Check sheet for the modelled part. Datum: model origin and axes. Units: mm. Round coordinates to 2 decimals unless told otherwise and drop trailing zeros. Write each loop counter-clockwise with the first axis right and the second up, starting at its lowest first coordinate (ties: lowest second). Pieces come first, ordered by that corner, then holes. Notation, with made-up numbers: (60, 69) - (98, 69) arc R26 ccw to (98, 101) - close; hole circle Ø5 at (17.5, 58.25). An arc over 180 degrees is marked (long way). Use one line per item in the form item = value. Start each with the question number.
1) Section check B-B (y = 1). Count the separate pieces of the cut face and the enclosed holes in it, then the cut area to 3 significant figures.
2) Scan lines: probe 1 along X at (y, z) = (2.8, 0); probe 2 along X at (y, z) = (4.25, 62); probe 3 along Z at (x, y) = (-38, 2.1). Record each from-to range of solid material in increasing order.
3) Section check A-A (z = -107). Record the boundary of the cut face in (x, y).
4) Gauge pin test, flat end, axial feed: P1, Ø3, axis at x = 27.5, z = -36, coming from the -Y side. Record the tip position at first contact, or that the pin passes through.
from build123d import *

# Parameters (mm, degrees)
SKETCH1_W           = 300
SKETCH1_H           = 300
BOSS_EXTRUDE1_DEPTH = 4.5
SKETCH3_W           = 4.9
SKETCH3_H           = 15.4
CUT_EXTRUDE1_DEPTH  = 213.179758695
SKETCH6_W           = 15
SKETCH6_H           = 25
CUT_EXTRUDE2_DEPTH  = 213.179758695
SKETCH7_W           = 4.9
SKETCH7_H           = 10.4
CUT_EXTRUDE3_DEPTH  = 213.179758695
SKETCH8_R           = 1.55
CUT_EXTRUDE4_DEPTH  = 213.179758695
FILLET1_R           = 5


with BuildPart() as part:
    # Sketch1 → Boss-Extrude1 (new body)
    with BuildSketch(Plane(origin=(0, 0, 0), x_dir=(1, 0, 0), z_dir=(0, 1, 0))):
        Rectangle(SKETCH1_W, SKETCH1_H)
    extrude(amount=BOSS_EXTRUDE1_DEPTH)

    # Sketch3 → Cut-Extrude1 (cut, through all)
    with BuildSketch(Plane.XZ):
        with Locations((18.5, -130.5)):
            Rectangle(SKETCH3_W, SKETCH3_H)
        with Locations((18.5, -110.5)):
            Rectangle(SKETCH3_W, SKETCH3_H)
        with Locations((-18.5, -110.5)):
            Rectangle(SKETCH3_W, SKETCH3_H)
        with Locations((-18.5, -130.5)):
            Rectangle(SKETCH3_W, SKETCH3_H)
    extrude(amount=-CUT_EXTRUDE1_DEPTH, mode=Mode.SUBTRACT)

    # Sketch6 → Cut-Extrude2 (cut, through all)
    with BuildSketch(Plane.XZ):
        with Locations((37.5, -72.5)):
            Rectangle(SKETCH6_W, SKETCH6_H)
        with Locations((37.5, 72.5)):
            Rectangle(SKETCH6_W, SKETCH6_H)
        with Locations((-37.5, 72.5)):
            Rectangle(SKETCH6_W, SKETCH6_H)
        with Locations((-37.5, -72.5)):
            Rectangle(SKETCH6_W, SKETCH6_H)
    extrude(amount=-CUT_EXTRUDE2_DEPTH, mode=Mode.SUBTRACT)

    # Sketch7 → Cut-Extrude3 (cut, through all)
    with BuildSketch(Plane.XZ):
        with Locations((14, 130)):
            Rectangle(SKETCH7_W, SKETCH7_H)
        with Locations((-14, 130)):
            Rectangle(SKETCH7_W, SKETCH7_H)
        with Locations((-14, 115)):
            Rectangle(SKETCH7_W, SKETCH7_H)
        with Locations((14, 115)):
            Rectangle(SKETCH7_W, SKETCH7_H)
    extrude(amount=-CUT_EXTRUDE3_DEPTH, mode=Mode.SUBTRACT)

    # Sketch8 → Cut-Extrude4 (cut, through all)
    with BuildSketch(Plane.XZ):
        with Locations(Location((70, 0, 0), (0, 0, 270))):
            Circle(SKETCH8_R)
        with Locations(Location((-70, 0, 0), (0, 0, 90))):
            Circle(SKETCH8_R)
    extrude(amount=-CUT_EXTRUDE4_DEPTH, mode=Mode.SUBTRACT)

    # Fillet1
    fillet1_edges = [part.edges().sort_by_distance(p)[0] for p in [
        (150, 2.25, 150),
        (-150, 2.25, 150),
        (-150, 2.25, -150),
        (150, 2.25, -150),
    ]]
    fillet(fillet1_edges, radius=FILLET1_R)


solid = part.part
Results are:
q1.separate_pieces = 1
q1.enclosed_holes = 14
q1.area = 88,000 mm²
q2.probe_1 = -150 to -71.55, -68.45 to 68.45, 71.55 to 150
q2.probe_2 = -150 to -45, -30 to 30, 45 to 150
q2.probe_3 = -150 to -85, -60 to 60, 85 to 150
q3.outline = (-150, 0) - (-20.95, 0) - (-20.95, 4.5) - (-150, 4.5) - close; (-16.05, 0) - (16.05, 0) - (16.05, 4.5) - (-16.05, 4.5) - close; (20.95, 0) - (150, 0) - (150, 4.5) - (20.95, 4.5) - close
q4.P1 = 0
